Drawing for the job (mm, zero at the part's lowest x, y, z). Give positions to 0.01 mm unless a question says otherwise; leave off trailing zeros. Loops run counter-clockwise (first coordinate to the right, second up) from the corner with the lowest first, then second, coordinate; pieces in that order, holes last. Notation, with made-up numbers: (23.25, 18) -> (61.25, 18) arc R22 ccw to (61.25, 57) -> close; hole circle Ø6 at (28.5, 47.5). An arc over 180 degrees is marked (long way). Write item = value, one per line.
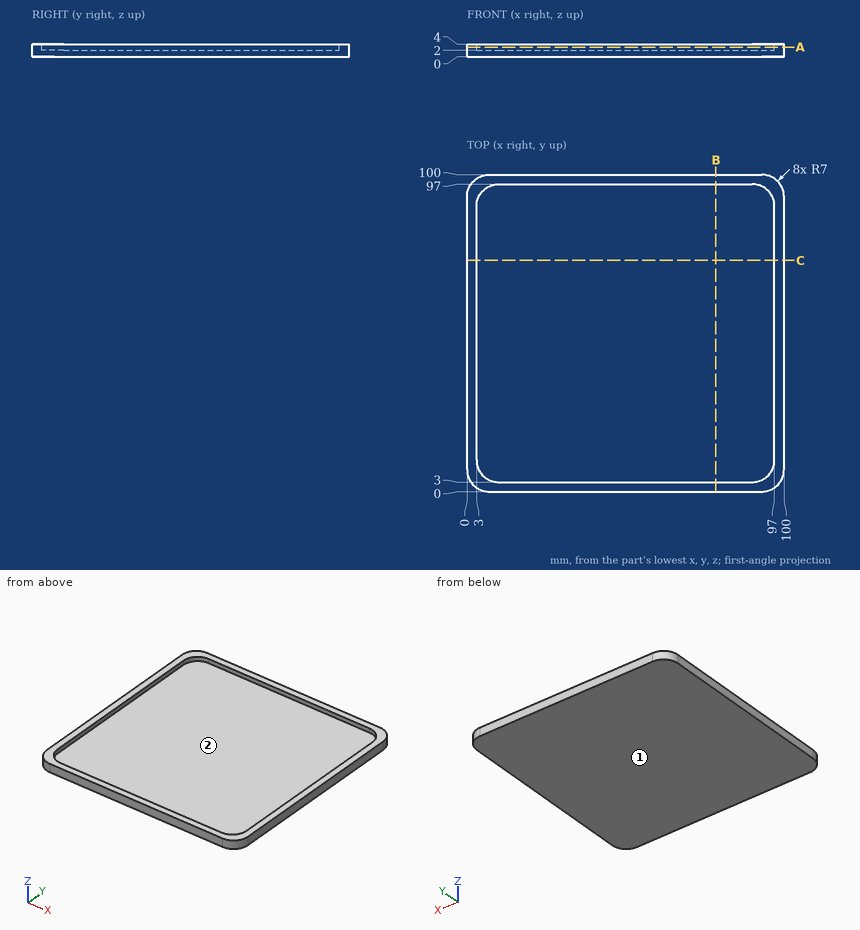
1) Drill centre lines: line 1 along Y through (x, z) = (48.5, 2.7); line 2 along Z through (x, y) = (74.5, 53.5). Where is each one in solid material? Low to high. Write a range as [from, to].
Resolved:
line_1 = [0, 3], [97, 100]
line_2 = [0, 2]
2) Slice it at A-A, the plane z = 3. List the corners of the cut face in (x, y), and give its area (3 significant figures).
Resolved:
outline = (0, 7) arc R7 ccw to (7, 0) -> (93, 0) arc R7 ccw to (100, 7) -> (100, 93) arc R7 ccw to (93, 100) -> (7, 100) arc R7 ccw to (0, 93) -> close; hole (3, 10) arc R7 ccw to (10, 3) -> (90, 3) arc R7 ccw to (97, 10) -> (97, 90) arc R7 ccw to (90, 97) -> (10, 97) arc R7 ccw to (3, 90) -> close
area = 1,160 mm²
3) Drop flat-ended pins along their axis: P1, Ø1.6, axis at x = 31.5, z = 2.5, coming from the -Y side; P2, Ø4, axis at x = 71.5, y = 78.5, coming from the +Z side. Give the stop position or say it passes through.
Resolved:
P1 = 0
P2 = 2
4) Pull direction Y, two halves, no side cores. Call the marked faces 1 and 2: pulls with the +Y half, pulls with the -Y half, needs draft (parallel to the pull), parting line crosses it, or undercut.
Resolved:
face_1 = needs draft
face_2 = undercut
5) Slice it at B-B, the plane x = 78.5. List the corners of the cut face in (y, z), and give its area (3 significant figures).
Resolved:
outline = (0, 0) -> (100, 0) -> (100, 4) -> (97, 4) -> (97, 2) -> (3, 2) -> (3, 4) -> (0, 4) -> close
area = 212 mm²
